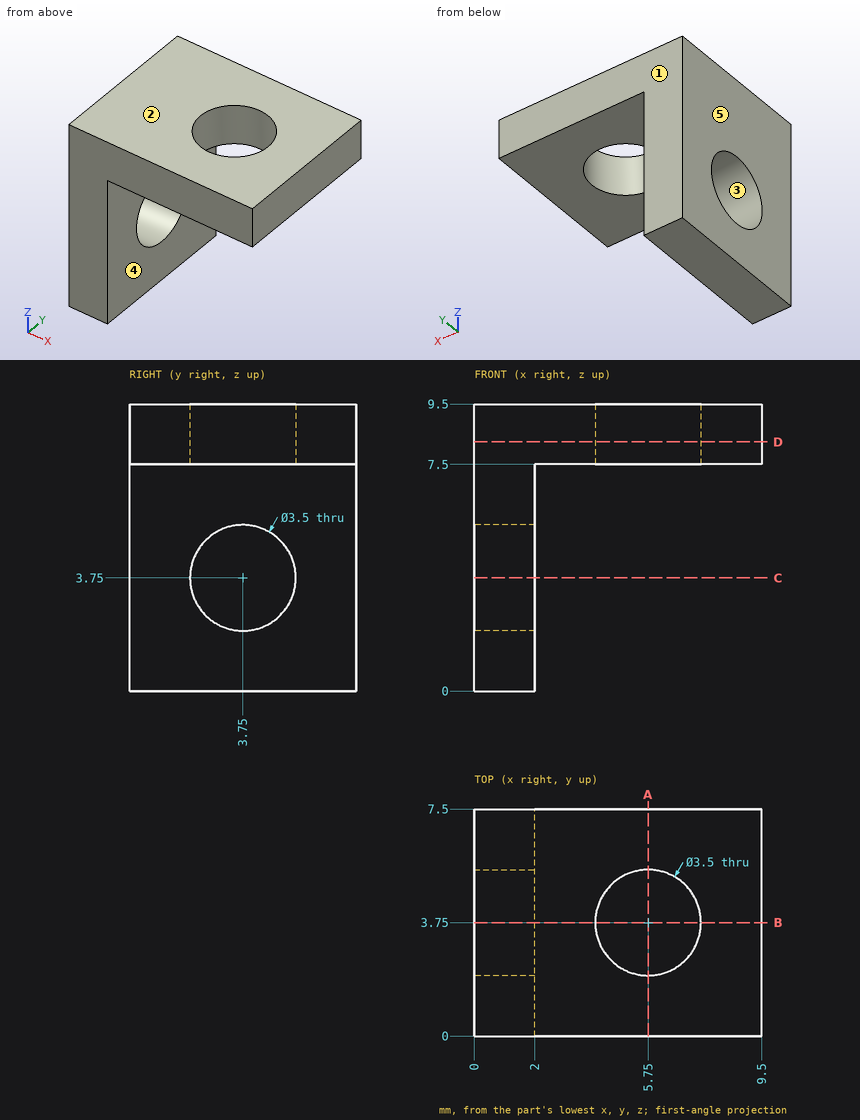
Can you work these out from the drawing? Everything is in mm from the part's minimum corner. A direction names the side the tool comes from. Coordinates: 2 decimals unless noted, no trailing zeros. Loops run counter-clockwise (first coordinate to the right, second up) from the corner with the lowest first, then second, coordinate; pieces in that order, holes last. Notation, with made-up numbers: M -32,56 L -24,56 A24 ccw -24,95 Z; hole C 17.25,-36.75 d6. An arc over 180 degrees is marked long. One line per item, written item: value.
1. Imagine slicing it at B-B (y = 3.75). List the corners of the cut face in (x, z) for me.
Geometry says:
outline: M 0,0 L 2,0 L 2,2 L 0,2 Z; M 0,5.5 L 2,5.5 L 2,7.5 L 4,7.5 L 4,9.5 L 0,9.5 Z; M 7.5,7.5 L 9.5,7.5 L 9.5,9.5 L 7.5,9.5 Z
2. Imagine slicing it at A-A (x = 5.75). List the corners of the cut face in (y, z) for me.
Geometry says:
outline: M 0,7.5 L 2,7.5 L 2,9.5 L 0,9.5 Z; M 5.5,7.5 L 7.5,7.5 L 7.5,9.5 L 5.5,9.5 Z
3. Thinking about a two-plate mould opening in Z: for the marked faces 1, 2 and 3, which applies, +Z half, -Z half, draft (parallel to the pull), parting line (faces both ways), or undercut?
Geometry says:
face 1: draft
face 2: +Z half
face 3: undercut
4. Please list where these lines run through material, in increasing order: probe 1 along Z at (x, y) = (0.7, 3.75); probe 2 along Y at (x, z) = (5.75, 8.05); probe 3 along X at (y, z) = (1.5, 7).
Geometry says:
probe 1: z = 0 to 2, 5.5 to 9.5
probe 2: y = 0 to 2, 5.5 to 7.5
probe 3: x = 0 to 2
5. Will these pins go through, and if not, where does the flat tip stop? pin 1 Ø4 at (y, z) = (4.5, 4.5) entering from +X; pin 2 Ø4 at (x, y) = (6.5, 3) entering from -Z.
Geometry says:
pin 1: stops at x = 2
pin 2: stops at z = 7.5
6. Imagine slicing it at D-D (z = 8.25). List the corners of the cut face in (x, y) for me.
Geometry says:
outline: M 0,0 L 9.5,0 L 9.5,7.5 L 0,7.5 Z; hole C 5.75,3.75 d3.5
7. Imagine slicing it at C-C (z = 3.75). List the corners of the cut face in (x, y) for me.
Geometry says:
outline: M 0,0 L 2,0 L 2,2 L 0,2 Z; M 0,5.5 L 2,5.5 L 2,7.5 L 0,7.5 Z
8. On a 3-axis mill with a long thin cutter (end or side, diameter ignored), from which of +Z, -Z, +X, -X, +Y, -Y can I reach the whole of each face in a straight line? I mean the marked faces 4 and 5. Say none if no direction works.
Geometry says:
face 4: -Z, +X, +Y, -Y
face 5: +Z, -Z, -X, +Y, -Y
